Autodesk Fusion 360 part; units mm, degrees
sketch "Sketch1" plane through (0, 0, 0) normal (0, 1, 0) x (1, 0, 0)
  line L0 (-35.75, 41.5) -> (-33.75, 41.5)
  line L1 (-33.75, 41.5) -> (-33.75, -41.5)
  line L2 (-33.75, -41.5) -> (33.75, -41.5)
  line L3 (33.75, -41.5) -> (33.75, 41.5)
  line L4 (33.75, 41.5) -> (35.75, 41.5)
  line L5 (35.75, 41.5) -> (35.75, -43.5)
  line L6 (35.75, -43.5) -> (-35.75, -43.5)
  line L7 (-35.75, -43.5) -> (-35.75, 41.5)
  dimension "d1" = 2
  dimension "d2" = 2
  dimension "d3" = 2
  dimension "d4" = 67.5
  dimension "d5" = 83
  dimension "d6" = 33.75
  dimension "d7" = 41.5
extrude "Extrude1" add sketch "Sketch1" along normal blind 5.1
sketch "Sketch2" plane through (0, 5.1, 0) normal (0, 1, 0) x (-1, 0, 0)
  line L0 (35.75, 43.5) -> (-35.75, 43.5)
  line L1 (-35.75, 43.5) -> (-35.75, -41.5)
  line L2 (-35.75, -41.5) -> (-33.75, -41.5)
  line L3 (-33.75, -41.5) -> (-33.75, 41.5)
  line L4 (-33.75, 41.5) -> (33.75, 41.5)
  line L5 (33.75, 41.5) -> (33.75, -41.5)
  line L6 (33.75, -41.5) -> (35.75, -41.5)
  line L7 (35.75, -41.5) -> (35.75, 43.5)
  line L8 (35.75, 43.5) -> (-35.75, 43.5)
  line L9 (-35.75, 43.5) -> (-35.75, -41.5)
  line L10 (-35.75, -41.5) -> (35.75, -41.5)
  line L11 (35.75, -41.5) -> (35.75, 43.5)
extrude "Extrude2" add sketch "Sketch2" along normal blind 2.5
equation "d2 = d1"
equation "d3 = d1"
equation "d4 = 60 mm + 6 mm + 1.5 mm"
equation "d5 = 80 mm + 3 mm"
equation "d6 = d4 / 2"
equation "d7 = d5 / 2"
Can you work these out from the model? Positions are in its coordinate system, mm. A direction names the side the tool comes from. Give positions to 0.01 mm unless a question says otherwise; leave off trailing zeros. Loops run counter-clockwise (first coordinate to the right, second up) from the corner with the lowest first, then second, coordinate; pieces in that order, holes last. Notation, with made-up numbers: M 26,86 L 35,86 A21 ccw 35,102 Z; hole C 11,7.5 d1. An arc over 180 degrees is marked long. Use CSV: the item, a comma, the result in double quotes. Start each with the question number.
1. For P1, Ø2, axis at x = -13, y = 2.5, coming from the -Z side; P2, Ø20, axis at x = -9.5, z = 2.5, coming from the -Y side, each with a flat end and sliding along its axis, tell me the tip position at first contact or that it passes through.
2. If I drill on L1, parallel to X at y = 1.25, z = -3; L2, parallel to Z at x = 26.5, y = 2.75; L3, parallel to Y at x = 2, z = 16.5, over which ranges is the centre line in solid material (lowest first)?
3. On a 3-axis mill with a long thin cutter (end or side, diameter ignored), from which of +Z, -Z, +X, -X, +Y, -Y can I reach the whole of each face in a straight line? I mean faces 1 (the face through (0, 6, -41.5)), 2 (the face through (0, 3, 41.5)). Say none if no direction works.
4. Imagine slicing it at B-B, the plane x = -24.5. Write out the boundary of the cut face in (y, z), plus the area to 3 significant figures.
5. Imagine slicing it at C-C, the plane z = 34. Write out the boundary of the cut face in (x, y).
6. Imagine slicing it at A-A, the plane y = 1.5. Write out the boundary of the cut face in (x, z).
7. If we mould it in two halves opening along X, with no side actions, what happens to faces 3 (the face through (0, 5.1, 1)), 4 (the face through (1, 4, 43.5)), 5 (the face through (-35.75, 4, 2)), 6 (the face through (35.75, 4, 0))? For each: released by +X, released by -X, zero draft, split by the parting line, or undercut.
Response values:
1,P1,"z = 41.5"
1,P2,"y = 5.1"
2,L1,"-35.75 to -33.75, 33.75 to 35.75"
2,L2,"41.5 to 43.5"
2,L3,"5.1 to 7.6"
3,face 1,"-Z, +X, -X, +Y, -Y"
3,face 2,"-Z, -Y"
4,outline,"M 0,41.5 L 5.1,41.5 L 5.1,-41.5 L 7.6,-41.5 L 7.6,43.5 L 0,43.5 Z"
4,area,"223 mm^2"
5,outline,"M -35.75,0 L -33.75,0 L -33.75,5.1 L 33.75,5.1 L 33.75,0 L 35.75,0 L 35.75,7.6 L -35.75,7.6 Z"
6,outline,"M -35.75,-41.5 L -33.75,-41.5 L -33.75,41.5 L 33.75,41.5 L 33.75,-41.5 L 35.75,-41.5 L 35.75,43.5 L -35.75,43.5 Z"
7,face 3,"undercut"
7,face 4,"zero draft"
7,face 5,"released by -X"
7,face 6,"released by +X"
